from build123d import *

# Parameters (mm, degrees)
F0_R     = 3.6
F0_R_2   = 11.1
F1_DEPTH = 6.5


with BuildPart() as f1:
    # F0 (on Top) → F1 (new body)
    with BuildSketch(Plane.XY):
        with BuildLine():
            ThreePointArc((12.7551052803, 5.7712467707), (13.2775282625, 2.8640474895), (14, 0))
            ThreePointArc((14, 0), (13.6852379213, 2.951993062), (12.7551052803, 5.7712467707))
        make_face()
        with BuildLine():
            ThreePointArc((12.7551052803, 5.7712467707), (13.6852379213, 2.951993062), (14, 0))
            ThreePointArc((14, 0), (13.6843771554, -2.9559806947), (12.7517397332, -5.7786792415))
            ThreePointArc((12.7517397332, -5.7786792415), (12.3951684194, -9.0411992807), (12.2812401035, -12.3211688608))
            ThreePointArc((12.2812401035, -12.3211688608), (27.4116387343, -15.2593204889), (40.5084826052, -23.3854744583))
            ThreePointArc((40.5084826052, -23.3854744583), (47.2547330266, -0.2211970993), (41.2789992988, 23.1537092477))
            ThreePointArc((41.2789992988, 23.1537092477), (27.7803945414, 15.1065071257), (12.3211688608, 12.2812401035))
            ThreePointArc((12.3211688608, 12.2812401035), (12.4134187433, 9.0179300915), (12.7551052803, 5.7712467707))
        make_face()
        with Locations((36.3028572677, -11.9313535626)):
            Circle(F0_R, mode=Mode.SUBTRACT)
        with Locations((39.9324558712, 0)):
            Circle(F0_R, mode=Mode.SUBTRACT)
        with Locations((36.3028572677, 11.9313535626)):
            Circle(F0_R, mode=Mode.SUBTRACT)
        with BuildLine():
            ThreePointArc((12.7517397332, -5.7786792415), (13.2793138092, -2.8684824171), (14, 0))
            ThreePointArc((14, 0), (13.2775282625, 2.8640474895), (12.7551052803, 5.7712467707))
            ThreePointArc((12.7551052803, 5.7712467707), (9.9023791422, 9.8966098905), (5.7786792415, 12.7517397332))
            ThreePointArc((5.7786792415, 12.7517397332), (2.8684824171, 13.2793138092), (0, 14))
            ThreePointArc((0, 14), (-2.8640474895, 13.2775282625), (-5.7712467707, 12.7551052803))
            ThreePointArc((-5.7712467707, 12.7551052803), (-9.8966098905, 9.9023791422), (-12.7517397332, 5.7786792415))
            ThreePointArc((-12.7517397332, 5.7786792415), (-13.2793138092, 2.8684824171), (-14, 0))
            ThreePointArc((-14, 0), (-13.2775282625, -2.8640474895), (-12.7551052803, -5.7712467707))
            ThreePointArc((-12.7551052803, -5.7712467707), (-9.9023791422, -9.8966098905), (-5.7786792415, -12.7517397332))
            ThreePointArc((-5.7786792415, -12.7517397332), (-2.8684824171, -13.2793138092), (0, -14))
            ThreePointArc((0, -14), (2.8640474895, -13.2775282625), (5.7712467707, -12.7551052803))
            ThreePointArc((5.7712467707, -12.7551052803), (9.8966098905, -9.9023791422), (12.7517397332, -5.7786792415))
        make_face()
        Circle(F0_R_2, mode=Mode.SUBTRACT)
        with BuildLine():
            ThreePointArc((12.7517397332, -5.7786792415), (13.6843771554, -2.9559806947), (14, 0))
            ThreePointArc((14, 0), (13.2793138092, -2.8684824171), (12.7517397332, -5.7786792415))
        make_face()
        with BuildLine():
            ThreePointArc((5.7786792415, 12.7517397332), (9.9023791422, 9.8966098905), (12.7551052803, 5.7712467707))
            ThreePointArc((12.7551052803, 5.7712467707), (12.4134187433, 9.0179300915), (12.3211688608, 12.2812401035))
            ThreePointArc((12.3211688608, 12.2812401035), (9.0411992807, 12.3951684194), (5.7786792415, 12.7517397332))
        make_face()
        with BuildLine():
            ThreePointArc((12.2812401035, -12.3211688608), (12.3951684194, -9.0411992807), (12.7517397332, -5.7786792415))
            ThreePointArc((12.7517397332, -5.7786792415), (9.8966098905, -9.9023791422), (5.7712467707, -12.7551052803))
            ThreePointArc((5.7712467707, -12.7551052803), (9.0179300915, -12.4134187433), (12.2812401035, -12.3211688608))
        make_face()
        with BuildLine():
            ThreePointArc((0, 14), (2.8684824171, 13.2793138092), (5.7786792415, 12.7517397332))
            ThreePointArc((5.7786792415, 12.7517397332), (2.9559806947, 13.6843771554), (0, 14))
        make_face()
        with BuildLine():
            ThreePointArc((0, 14), (2.9559806947, 13.6843771554), (5.7786792415, 12.7517397332))
            ThreePointArc((5.7786792415, 12.7517397332), (9.0411992807, 12.3951684194), (12.3211688608, 12.2812401035))
            ThreePointArc((12.3211688608, 12.2812401035), (15.2593204889, 27.4116387343), (23.3854744583, 40.5084826052))
            ThreePointArc((23.3854744583, 40.5084826052), (0.2211970993, 47.2547330266), (-23.1537092477, 41.2789992988))
            ThreePointArc((-23.1537092477, 41.2789992988), (-15.1065071257, 27.7803945414), (-12.2812401035, 12.3211688608))
            ThreePointArc((-12.2812401035, 12.3211688608), (-9.0179300915, 12.4134187433), (-5.7712467707, 12.7551052803))
            ThreePointArc((-5.7712467707, 12.7551052803), (-2.951993062, 13.6852379213), (0, 14))
        make_face()
        with Locations((-11.9313535626, 36.3028572677)):
            Circle(F0_R, mode=Mode.SUBTRACT)
        with Locations((0, 39.9324558712)):
            Circle(F0_R, mode=Mode.SUBTRACT)
        with Locations((11.9313535626, 36.3028572677)):
            Circle(F0_R, mode=Mode.SUBTRACT)
        with BuildLine():
            ThreePointArc((12.2812401035, -12.3211688608), (9.0179300915, -12.4134187433), (5.7712467707, -12.7551052803))
            ThreePointArc((5.7712467707, -12.7551052803), (2.951993062, -13.6852379213), (0, -14))
            ThreePointArc((0, -14), (-2.9559806947, -13.6843771554), (-5.7786792415, -12.7517397332))
            ThreePointArc((-5.7786792415, -12.7517397332), (-9.0411992807, -12.3951684194), (-12.3211688608, -12.2812401035))
            ThreePointArc((-12.3211688608, -12.2812401035), (-15.2593204889, -27.4116387343), (-23.3854744583, -40.5084826052))
            ThreePointArc((-23.3854744583, -40.5084826052), (-0.2211970993, -47.2547330266), (23.1537092477, -41.2789992988))
            ThreePointArc((23.1537092477, -41.2789992988), (15.1065071257, -27.7803945414), (12.2812401035, -12.3211688608))
        make_face()
        with Locations((-11.9313535626, -36.3028572677)):
            Circle(F0_R, mode=Mode.SUBTRACT)
        with Locations((0, -39.9324558712)):
            Circle(F0_R, mode=Mode.SUBTRACT)
        with Locations((11.9313535626, -36.3028572677)):
            Circle(F0_R, mode=Mode.SUBTRACT)
        with BuildLine():
            ThreePointArc((0, -14), (2.951993062, -13.6852379213), (5.7712467707, -12.7551052803))
            ThreePointArc((5.7712467707, -12.7551052803), (2.8640474895, -13.2775282625), (0, -14))
        make_face()
        with BuildLine():
            ThreePointArc((-5.7712467707, 12.7551052803), (-2.8640474895, 13.2775282625), (0, 14))
            ThreePointArc((0, 14), (-2.951993062, 13.6852379213), (-5.7712467707, 12.7551052803))
        make_face()
        with BuildLine():
            ThreePointArc((-5.7786792415, -12.7517397332), (-2.9559806947, -13.6843771554), (0, -14))
            ThreePointArc((0, -14), (-2.8684824171, -13.2793138092), (-5.7786792415, -12.7517397332))
        make_face()
        with BuildLine():
            ThreePointArc((-12.7517397332, 5.7786792415), (-9.8966098905, 9.9023791422), (-5.7712467707, 12.7551052803))
            ThreePointArc((-5.7712467707, 12.7551052803), (-9.0179300915, 12.4134187433), (-12.2812401035, 12.3211688608))
            ThreePointArc((-12.2812401035, 12.3211688608), (-12.3951684194, 9.0411992807), (-12.7517397332, 5.7786792415))
        make_face()
        with BuildLine():
            ThreePointArc((-12.3211688608, -12.2812401035), (-9.0411992807, -12.3951684194), (-5.7786792415, -12.7517397332))
            ThreePointArc((-5.7786792415, -12.7517397332), (-9.9023791422, -9.8966098905), (-12.7551052803, -5.7712467707))
            ThreePointArc((-12.7551052803, -5.7712467707), (-12.4134187433, -9.0179300915), (-12.3211688608, -12.2812401035))
        make_face()
        with BuildLine():
            ThreePointArc((-14, 0), (-13.2793138092, 2.8684824171), (-12.7517397332, 5.7786792415))
            ThreePointArc((-12.7517397332, 5.7786792415), (-13.6843771554, 2.9559806947), (-14, 0))
        make_face()
        with BuildLine():
            ThreePointArc((-14, 0), (-13.6843771554, 2.9559806947), (-12.7517397332, 5.7786792415))
            ThreePointArc((-12.7517397332, 5.7786792415), (-12.3951684194, 9.0411992807), (-12.2812401035, 12.3211688608))
            ThreePointArc((-12.2812401035, 12.3211688608), (-27.4116387343, 15.2593204889), (-40.5084826052, 23.3854744583))
            ThreePointArc((-40.5084826052, 23.3854744583), (-47.2547330266, 0.2211970993), (-41.2789992988, -23.1537092477))
            ThreePointArc((-41.2789992988, -23.1537092477), (-27.7803945414, -15.1065071257), (-12.3211688608, -12.2812401035))
            ThreePointArc((-12.3211688608, -12.2812401035), (-12.4134187433, -9.0179300915), (-12.7551052803, -5.7712467707))
            ThreePointArc((-12.7551052803, -5.7712467707), (-13.6852379213, -2.951993062), (-14, 0))
        make_face()
        with Locations((-36.3028572677, -11.9313535626)):
            Circle(F0_R, mode=Mode.SUBTRACT)
        with Locations((-39.9324558712, 0)):
            Circle(F0_R, mode=Mode.SUBTRACT)
        with Locations((-36.3028572677, 11.9313535626)):
            Circle(F0_R, mode=Mode.SUBTRACT)
        with BuildLine():
            ThreePointArc((-14, 0), (-13.6852379213, -2.951993062), (-12.7551052803, -5.7712467707))
            ThreePointArc((-12.7551052803, -5.7712467707), (-13.2775282625, -2.8640474895), (-14, 0))
        make_face()
    extrude(amount=F1_DEPTH)


solid = f1.part
Design review of the part built by this model. Coordinates are the model's own, in mm. A direction names the side the tool comes from. Give positions to 0.01 mm unless a question says otherwise; leave off trailing zeros. Order: outer loops, then holes, each group sorted by start corner. A loop starts at its lowest first (then second) coordinate and runs counter-clockwise, first axis right, second up.
1. Add section C-C, the plane z = 4.25. State how many separate pieces and enclosed holes the cut face has, then the cut area to 3 significant figures.
Solution:
separate pieces: 1
enclosed holes: 13
area: 4,140 mm2
2. For pin 1 Ø11.5 at (x, y) = (36.3, 11.93) entering from +Z; pin 2 Ø1.5 at (y, z) = (2.5, 1) entering from -X; pin 3 Ø2 at (x, z) = (31.5, 1.5) entering from -Y; pin 4 Ø2 at (x, z) = (-35.5, 6) entering from +Y, all flat-tipped, find the tip position at first contact; note any pin that passes through.
Solution:
pin 1: stops at z = 6.5
pin 2: stops at x = -47.2
pin 3: stops at y = -17.65
pin 4: stops at y = 20.17
3. Add section B-B, the plane y = 0. State the section outline as (x, z) points.
Solution:
outline: (-47.26, 0) - (-43.53, 0) - (-43.53, 6.5) - (-47.26, 6.5) - close; (-36.33, 0) - (-11.1, 0) - (-11.1, 6.5) - (-36.33, 6.5) - close; (11.1, 0) - (36.33, 0) - (36.33, 6.5) - (11.1, 6.5) - close; (43.53, 0) - (47.26, 0) - (47.26, 6.5) - (43.53, 6.5) - close
4. Mouldability with a two-part tool opening along X and no side actions: class faces 1 (the cylindrical face through (0.563, 47.248, 3.204)), 2 (the cylindrical face through (-39.9, -11.8, 3.2)), 3 (the flat face through (10, -10, 6.5)) as +X half, -X half, draft (parallel to the pull), parting line (faces both ways), or undercut.
Solution:
face 1: parting line
face 2: undercut
face 3: draft
5. To check wall thickness, follow L1, parallel to Y at x = 0, z = 2.5; L2, parallel to X at y = 3, z = 6; L3, parallel to X at y = 34.5, z = 5. State the ranges of each line that lie inside material, in increasing order.
Solution:
L1: y = -47.26 to -43.53, -36.33 to -11.1, 11.1 to 36.33, 43.53 to 47.26
L2: x = -47.12 to -41.92, -37.94 to -10.69, 10.69 to 37.94, 41.92 to 47.19
L3: x = -18.3 to -15.05, -8.82 to 8.82, 15.05 to 18.83
6. Add section A-A, the plane x = -1. State the section outline as (y, z) points.
Solution:
outline: (-47.24, 0) - (-43.39, 0) - (-43.39, 6.5) - (-47.24, 6.5) - close; (-36.47, 0) - (-11.05, 0) - (-11.05, 6.5) - (-36.47, 6.5) - close; (11.05, 0) - (36.47, 0) - (36.47, 6.5) - (11.05, 6.5) - close; (43.39, 0) - (47.26, 0) - (47.26, 6.5) - (43.39, 6.5) - close
7. Tool access review of faces 4 (the cylindrical face through (27.987, 15.185, 3.204)), 5 (the flat face through (10, -10, 0)): name each direction out of +Z, -Z, +X, -X, +Y, -Y from which nothing blocks a thin tool from reaching the whole face with its end or side.
Solution:
face 4: +Z, -Z
face 5: -Z, +X, -X, +Y, -Y
8. Add section D-D, the plane y = -17. State the section outline as (x, z) points, then the cut area to 3 significant figures.
Solution:
outline: (-44.2, 0) - (-32.11, 0) - (-32.11, 6.5) - (-44.2, 6.5) - close; (-12.63, 0) - (12.54, 0) - (12.54, 6.5) - (-12.63, 6.5) - close; (31.28, 0) - (43.77, 0) - (43.77, 6.5) - (31.28, 6.5) - close
area: 323 mm2
